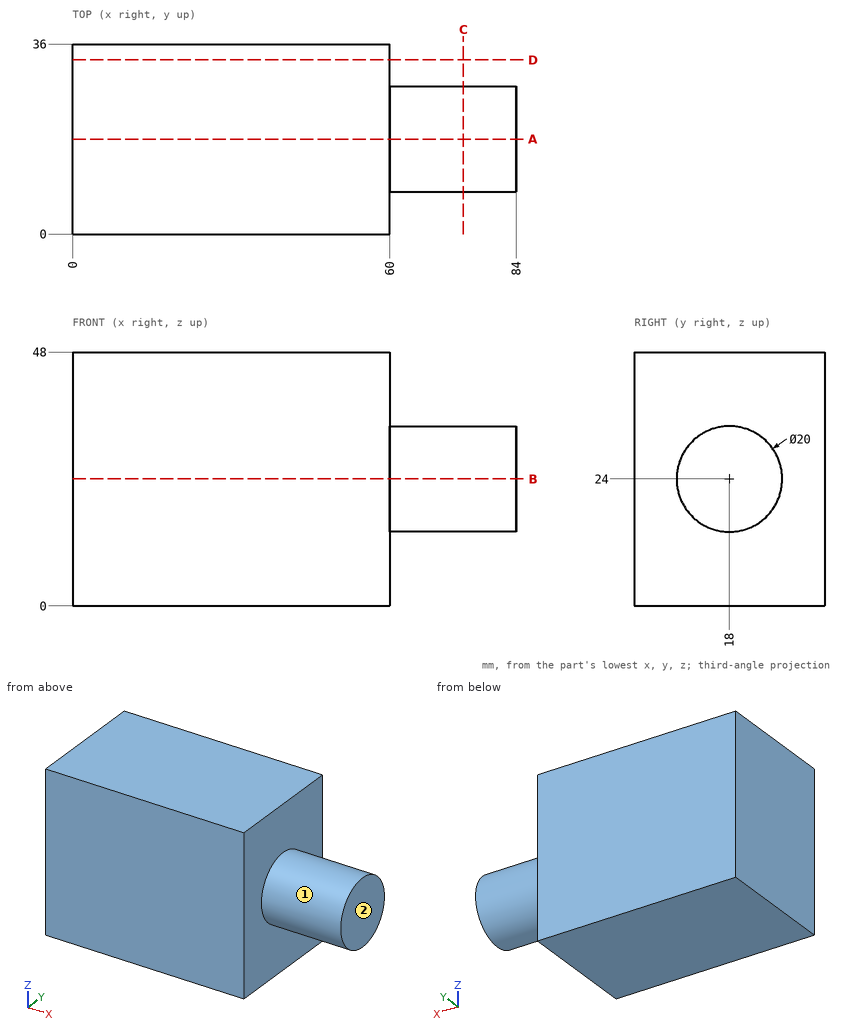
Here's the drawing with two shaded views (mm, measured from the low corner). I have some questions. A direction names the side the tool comes from. Give positions to 0.01 mm unless a question says otherwise; leave off trailing zeros. Loops run counter-clockwise (first coordinate to the right, second up) from the corner with the lowest first, then second, coordinate; pieces in that order, holes last. Notation, with made-up numbers: M -2,54 L 10,54 A30 cw 10,82 Z; hole C 77.25,89.25 d3. An arc over 180 degrees is marked long. One line per item, written item: value.
(1) Suppose I cut it at D-D on y = 33. List the corners of the cut face in (x, z) for me, plus the area to 3 significant figures.
Returned:
outline: M 0,0 L 60,0 L 60,48 L 0,48 Z
area: 2,880 mm^2
(2) Suppose I cut it at A-A on y = 18. List the corners of the cut face in (x, z) for me, plus the area to 3 significant figures.
Returned:
outline: M 0,0 L 60,0 L 60,14 L 84,14 L 84,34 L 60,34 L 60,48 L 0,48 Z
area: 3,360 mm^2
(3) I need wall thicknesses on line 1 (X direction, y = 29, z = 18); line 2 (Z direction, x = 69, y = 12.5); line 3 (Z direction, x = 76, y = 9.5). Which ranges of each line are inside material? Lowest first, please.
Returned:
line 1: 0 to 60
line 2: 15.65 to 32.35
line 3: 18.73 to 29.27
(4) Suppose I cut it at B-B on z = 24. List the corners of the cut face in (x, y) for me, plus the area to 3 significant figures.
Returned:
outline: M 0,0 L 60,0 L 60,8 L 84,8 L 84,28 L 60,28 L 60,36 L 0,36 Z
area: 2,640 mm^2
(5) Will these pins go through, and if not, where does the flat tip stop? pin 1 (6 mm diameter, centred on x = 65, z = 20.5, fed in from -Y); pin 2 (6 mm diameter, centred on y = 13, z = 38.5, fed in from +X).
Returned:
pin 1: y = 8.01
pin 2: x = 60
(6) Suppose I cut it at C-C on x = 74. List the corners of the cut face in (y, z) for me.
Returned:
outline: C 18,24 d20
(7) Which directions (+Z, -Z, +X, -X, +Y, -Y) give clear straight access to the entire face, cutting with the end or side of a thin tool? Please do the marked faces 1 and 2.
Returned:
face 1: +X
face 2: +Z, -Z, +X, +Y, -Y
